```python
from build123d import *

# Parameters (mm, degrees)
SKETCH1_W           = 30
SKETCH1_H           = 7.5
BOSS_EXTRUDE1_DEPTH = 5
SKETCH2_R           = 3.75
SKETCH2_R_2         = 2.5
BOSS_EXTRUDE2_DEPTH = 4
SKETCH3_R           = 1.75
CUT_EXTRUDE1_DEPTH  = 18.890290663
SKETCH4_R           = 2.5
CUT_EXTRUDE3_DEPTH  = 4
SKETCH5_R           = 1
CUT_EXTRUDE4_DEPTH  = 10
CUT_EXTRUDE5_START  = -10
SKETCH6_R           = 1
CUT_EXTRUDE5_DEPTH  = 10


with BuildPart() as part:
    # Sketch1 → Boss-Extrude1 (new body)
    with BuildSketch(Plane(origin=(0, 0, 0), x_dir=(1, 0, 0), z_dir=(0, 1, 0))):
        Rectangle(SKETCH1_W, SKETCH1_H)
    extrude(amount=BOSS_EXTRUDE1_DEPTH)

    # Sketch2 → Boss-Extrude2 (add)
    with BuildSketch(Plane(origin=(0, 5, 0), x_dir=(1, 0, 0), z_dir=(0, 1, 0))):
        with Locations(Location((0, 0, 0), (0, 0, 270))):
            Circle(SKETCH2_R)
        with Locations(Location((0, 0, 0), (0, 0, 270))):
            Circle(SKETCH2_R_2, mode=Mode.SUBTRACT)
    extrude(amount=BOSS_EXTRUDE2_DEPTH)

    # Sketch3 → Cut-Extrude1 (cut, through all)
    with BuildSketch(Plane.XZ):
        with Locations(Location((0, 0, 0), (0, 0, 270))):
            Circle(SKETCH3_R)
    extrude(amount=-CUT_EXTRUDE1_DEPTH, mode=Mode.SUBTRACT)

    # Sketch4 → Cut-Extrude3 (cut)
    with BuildSketch(Plane(origin=(0, 0, 0), x_dir=(-1, 0, 0), z_dir=(0, -1, 0))):
        with Locations(Location((0, 0, 0), (0, 0, 270))):
            Circle(SKETCH4_R)
    extrude(amount=-CUT_EXTRUDE3_DEPTH, mode=Mode.SUBTRACT)

    # Sketch5 → Cut-Extrude4 (cut)
    with BuildSketch(Plane(origin=(15, 0, 0), x_dir=(0, 0, -1), z_dir=(1, 0, 0))):
        with Locations((-0.25, 2.5)):
            Circle(SKETCH5_R)
    extrude(amount=-CUT_EXTRUDE4_DEPTH, mode=Mode.SUBTRACT)

    # Sketch6 → Cut-Extrude5 (cut)
    with BuildSketch(Plane.ZY.offset(15).offset(CUT_EXTRUDE5_START)):
        with Locations(Location((0.25, 2.5, 0), (0, 0, 180))):
            Circle(SKETCH6_R)
    extrude(amount=CUT_EXTRUDE5_DEPTH, mode=Mode.SUBTRACT)


solid = part.part
```
Geometry check sheet. Reference: the model listing, model coordinates, mm. A direction names the side the tool comes from. Give positions to 0.01 mm unless a question says otherwise; leave off trailing zeros. Loops run counter-clockwise (first coordinate to the right, second up) from the corner with the lowest first, then second, coordinate; pieces in that order, holes last. Notation, with made-up numbers: M 30.25,-2.75 L 87.25,-2.75 A27 ccw 87.25,35.25 Z; hole C 81,9 d8. An arc over 180 degrees is marked long. Write item = value, one per line. Start each with the question number.
1. Section check B-B, the plane y = 2.5. Enter the section's corners in (x, z).
2. Tool access check on faces 1 (the face through (10.07, 3.49, 0.38)), 2 (the face through (-2, 4, 1)), 3 (the face through (-9.93, 3.476, 0.467)), 4 (the face through (-2.44, 6.97, -0.54)). Record the directions out of +Z, -Z, +X, -X, +Y, -Y that give a thin tool (end or side, any length) a straight path to the whole face; none if there is none.
3. Section check D-D, the plane y = 5.5. Enter the section's corners in (x, z).
4. Thickness scan on probe 1 along Z at (x, y) = (-9, 2.5); probe 2 along X at (y, z) = (7, 0); probe 3 along Y at (x, z) = (7, 0.25). Record the ranges inside material, lowest first.
5. Draft check along Z on faces 5 (the face through (-5, 2, 0)), 6 (the face through (0, 0, -3)), 7 (the face through (0.165, 6.972, -3.746)). Enter one of: +Z half, -Z half, draft (parallel to the pull), parting line (faces both ways), or undercut.
6. Section check C-C, the plane z = 0. Enter the section's corners in (x, y).
7. Section check A-A, the plane x = 11.75. Enter the section's corners in (y, z).
8. Go/stop test with flat-tipped pins: P1, Ø2.5, axis at x = 0, z = 1, coming from the +Y side; P2, Ø1.6, axis at y = 2.5, z = 0.25, coming from the -X side; P3, Ø2, axis at y = 7.5, z = 0, coming from the +X side. Record where each tip stops, or that it passes through.
Values follow:
q1.outline = M -15,-3.75 L 15,-3.75 L 15,-0.75 L 5,-0.75 L 5,1.25 L 15,1.25 L 15,3.75 L -15,3.75 L -15,1.25 L -5,1.25 L -5,-0.75 L -15,-0.75 Z; hole C 0,0 d5
q2.face_1 = +X
q2.face_2 = -Y
q2.face_3 = -X
q2.face_4 = +Y
q3.outline = C 0,0 d7.5; hole C 0,0 d5
q4.probe_1 = -3.75 to -0.75, 1.25 to 3.75
q4.probe_2 = -3.75 to -2.5, 2.5 to 3.75
q4.probe_3 = 0 to 1.5, 3.5 to 5
q5.face_5 = undercut
q5.face_6 = draft
q5.face_7 = parting line
q6.outline = M -15,0 L -2.5,0 L -2.5,4 L -1.75,4 L -1.75,5 L -2.5,5 L -2.5,9 L -3.75,9 L -3.75,5 L -15,5 L -15,3.47 L -5,3.47 L -5,1.53 L -15,1.53 Z; M 1.75,4 L 2.5,4 L 2.5,0 L 15,0 L 15,1.53 L 5,1.53 L 5,3.47 L 15,3.47 L 15,5 L 3.75,5 L 3.75,9 L 2.5,9 L 2.5,5 L 1.75,5 Z
q7.outline = M 0,-3.75 L 5,-3.75 L 5,3.75 L 0,3.75 Z; hole C 2.5,0.25 d2
q8.P1 = 5
q8.P2 = -5
q8.P3 = 3.75
